Input: dimensioned drawing with shaded views. Units: mm. Origin: part minimum x, y, z. A direction names the side the tool comes from. Give positions to 0.01 mm unless a question says otherwise; leave off trailing zeros. Order: outer loops, then holes, each group sorted by start corner. A loop starts at its lowest first (then second) coordinate and runs counter-clockwise, first axis right, second up. Notation, with made-up numbers: (43.5, -38.75) -> (59.5, -38.75) arc R22 cw to (59.5, -31.75) -> close; hole circle Ø7 at (80.5, 33.25). An arc over 180 degrees is marked (long way). Use CSV: the item, a comma, the result in double quotes.
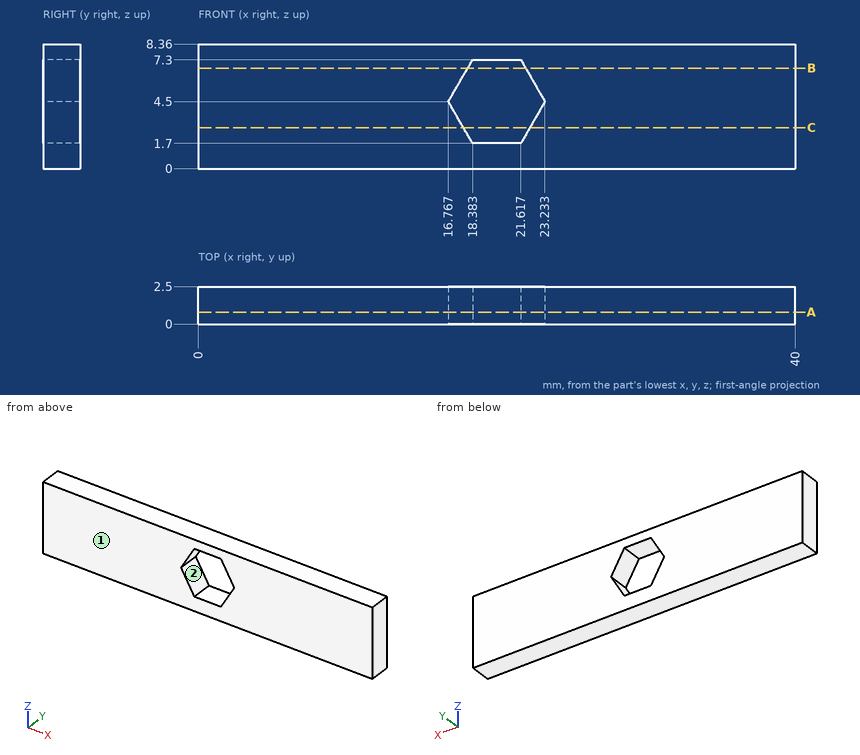
1. Section query A-A on y = 0.8. Return loops of the section in (x, z).
Answer below:
outline,"(0, 0) -> (40, 0) -> (40, 8.36) -> (0, 8.36) -> close; hole (16.77, 4.5) -> (18.38, 1.7) -> (21.62, 1.7) -> (23.23, 4.5) -> (21.62, 7.3) -> (18.38, 7.3) -> close"
2. Section query B-B on z = 6.75. Return loops of the section in (x, y).
Answer below:
outline,"(0, 0) -> (18.07, 0) -> (18.07, 2.5) -> (0, 2.5) -> close; (21.93, 0) -> (40, 0) -> (40, 2.5) -> (21.93, 2.5) -> close"
3. Access query for the marked faces 1 and 2. Directions: +Z, -Z, +X, -X, +Y, -Y. A direction counts if a zero-diameter tool reaches every point of the face in a straight line with its end or side. Return the directions, or none.
Answer below:
face 1,"+Z, -Z, +X, -X, -Y"
face 2,"+Y, -Y"
4. Ray query, line 1 along Z through (x, y) = (21, 2.3); line 2 along X through (y, z) = (0.65, 5) (1 decimal); line 3 along Z through (x, y) = (22.5, 1.9). Return the intervals inside material, ascending.
Answer below:
line 1,"z = 0 to 1.7, 7.3 to 8.36"
line 2,"x = 0 to 17.1, 22.9 to 40"
line 3,"z = 0 to 3.23, 5.77 to 8.36"
5. Section query C-C on z = 2.75. Return loops of the section in (x, y).
Answer below:
outline,"(0, 0) -> (17.78, 0) -> (17.78, 2.5) -> (0, 2.5) -> close; (22.22, 0) -> (40, 0) -> (40, 2.5) -> (22.22, 2.5) -> close"
